from build123d import *

# Parameters (mm, degrees)
SKETCH1_W               = 100
SKETCH1_H               = 70
BOSS_EXTRUDE1_DEPTH     = 6
SKETCH2_W               = 100
SKETCH2_H               = 6
BOSS_EXTRUDE2_DEPTH     = 50
CUT_EXTRUDE1_DEPTH      = 103.645019363
CUT_EXTRUDE1_DEPTH_BACK = 103.645019363
SKETCH3_R               = 1.5
SKETCH3_R_2             = 2
CUT_EXTRUDE2_DEPTH      = 103.645019363
CUT_EXTRUDE2_DEPTH_BACK = 103.645019363
CUT_EXTRUDE3_DEPTH      = 103.645019363
CUT_EXTRUDE4_DEPTH      = 103.645019363
CUT_EXTRUDE4_DEPTH_BACK = 103.645019363
CUT_EXTRUDE5_DEPTH      = 103.645019363
CUT_EXTRUDE5_DEPTH_BACK = 103.645019363
SKETCH9_W               = 15
SKETCH9_H               = 3.5
BOSS_EXTRUDE3_DEPTH     = 10
CUT_EXTRUDE8_START      = -3.5
SKETCH11_R              = 2
CUT_EXTRUDE8_DEPTH      = 12
FILLET1_R               = 5
FILLET2_R               = 5
FILLET3_R               = 5
FILLET4_R               = 5
CUT_EXTRUDE9_DEPTH      = 103.645019363
SKETCH14_R              = 5
CUT_EXTRUDE10_DEPTH     = 3
CUT_EXTRUDE11_START     = -3
SKETCH15_R              = 5
CUT_EXTRUDE11_DEPTH     = 3
SKETCH16_R              = 5
CUT_EXTRUDE12_DEPTH     = 3
CUT_EXTRUDE13_START     = -3
SKETCH17_R              = 5
CUT_EXTRUDE13_DEPTH     = 3


with BuildPart() as part:
    # Sketch1 → Boss-Extrude1 (new body)
    with BuildSketch(Plane(origin=(0, 0, 0), x_dir=(1, 0, 0), z_dir=(0, 1, 0))):
        Rectangle(SKETCH1_W, SKETCH1_H)
    extrude(amount=BOSS_EXTRUDE1_DEPTH)

    # Sketch2 → Boss-Extrude2 (add)
    with BuildSketch(Plane(origin=(0, 6, 0), x_dir=(1, 0, 0), z_dir=(0, 1, 0))):
        with Locations((0, 32)):
            Rectangle(SKETCH2_W, SKETCH2_H)
        with Locations((0, -32)):
            Rectangle(SKETCH2_W, SKETCH2_H)
    extrude(amount=BOSS_EXTRUDE2_DEPTH)

    # Sketch3 → Cut-Extrude1 (cut, two sides: drawn at the far end of the back side and taken through both)
    with BuildSketch(Plane.XY.offset(35).offset(-CUT_EXTRUDE1_DEPTH_BACK)):
        with Locations((-35, 11)):
            Circle(SKETCH3_R)
        with Locations((25, 11)):
            Circle(SKETCH3_R_2)
    extrude(amount=CUT_EXTRUDE1_DEPTH + CUT_EXTRUDE1_DEPTH_BACK, mode=Mode.SUBTRACT)

    # Sketch4 → Cut-Extrude2 (cut, two sides: drawn at the far end of the back side and taken through both)
    with BuildSketch(Plane.XY.offset(35).offset(-CUT_EXTRUDE2_DEPTH_BACK)):
        Polygon((-50, 25), (3.693575035, 56), (-50, 56), align=None)
    extrude(amount=CUT_EXTRUDE2_DEPTH + CUT_EXTRUDE2_DEPTH_BACK, mode=Mode.SUBTRACT)

    # Sketch5 → Cut-Extrude3 (cut, through all)
    with BuildSketch(Plane.XY.offset(35)):
        Polygon((26.846787517, 56), (50, 28), (50, 56), align=None)
    extrude(amount=-CUT_EXTRUDE3_DEPTH, mode=Mode.SUBTRACT)

    # Sketch6 → Cut-Extrude4 (cut, two sides: drawn at the far end of the back side and taken through both)
    with BuildSketch(Plane.XY.offset(35).offset(-CUT_EXTRUDE4_DEPTH_BACK)):
        Polygon((16.600357162, 47.527222171), (39.753569645, 19.527222171), (47.460108019, 25.899762189), (24.306895537, 53.899762189), align=None)
    extrude(amount=CUT_EXTRUDE4_DEPTH + CUT_EXTRUDE4_DEPTH_BACK, mode=Mode.SUBTRACT)

    # Sketch7 → Cut-Extrude5 (cut, two sides: drawn at the far end of the back side and taken through both)
    with BuildSketch(Plane.XY.offset(35).offset(-CUT_EXTRUDE5_DEPTH_BACK)):
        Polygon((2.673241004, 38.01310693), (-4.304705141, 32.243040152), (11.948586847, 12.587358417), (18.926532993, 18.357425196), align=None)
        Polygon((-15.212346405, 34.449406206), (-22.19029255, 28.679339427), (-9.445212514, 13.266262678), (-2.467266369, 19.036329456), align=None)
    extrude(amount=CUT_EXTRUDE5_DEPTH + CUT_EXTRUDE5_DEPTH_BACK, mode=Mode.SUBTRACT)

    # Sketch9 → Boss-Extrude3 (add)
    with BuildSketch(Plane(origin=(0, 6, 0), x_dir=(1, 0, 0), z_dir=(0, 1, 0))):
        with Locations((-17.5, 4.25)):
            Rectangle(SKETCH9_W, SKETCH9_H)
        with Locations((-17.5, -4.25)):
            Rectangle(SKETCH9_W, SKETCH9_H)
    extrude(amount=BOSS_EXTRUDE3_DEPTH)

    # Sketch11 → Cut-Extrude8 (cut)
    with BuildSketch(Plane.XY.offset(-2.5).offset(CUT_EXTRUDE8_START)):
        with Locations((-17.5, 11)):
            Circle(SKETCH11_R)
    extrude(amount=CUT_EXTRUDE8_DEPTH, mode=Mode.SUBTRACT)

    # Fillet1
    fillet1_edges = [part.edges().sort_by_distance(p)[0] for p in [
        (-25, 16, -4.25),
    ]]
    fillet(fillet1_edges, radius=FILLET1_R)

    # Fillet2
    fillet2_edges = [part.edges().sort_by_distance(p)[0] for p in [
        (-10, 16, -4.25),
    ]]
    fillet(fillet2_edges, radius=FILLET2_R)

    # Fillet3
    fillet3_edges = [part.edges().sort_by_distance(p)[0] for p in [
        (-25, 16, 4.25),
    ]]
    fillet(fillet3_edges, radius=FILLET3_R)

    # Fillet4
    fillet4_edges = [part.edges().sort_by_distance(p)[0] for p in [
        (-10, 16, 4.25),
    ]]
    fillet(fillet4_edges, radius=FILLET4_R)

    # Sketch13 → Cut-Extrude9 (cut, through all)
    with BuildSketch(Plane(origin=(0, 0, -35), x_dir=(-1, 0, 0), z_dir=(0, 0, -1))):
        Polygon((-50, 12), (-39.487682116, 12), (-11.373066959, 46), (13.626933041, 46), (-3.693575035, 56), (-26.846787517, 56), (-50, 28), align=None)
    extrude(amount=-CUT_EXTRUDE9_DEPTH, mode=Mode.SUBTRACT)

    # Sketch14 → Cut-Extrude10 (cut)
    with BuildSketch(Plane.XY.offset(35)):
        with Locations((25, 11)):
            Circle(SKETCH14_R)
    extrude(amount=-CUT_EXTRUDE10_DEPTH, mode=Mode.SUBTRACT)

    # Sketch15 → Cut-Extrude11 (cut)
    with BuildSketch(Plane(origin=(0, 0, -35), x_dir=(-1, 0, 0), z_dir=(0, 0, -1)).offset(CUT_EXTRUDE11_START)):
        with Locations(Location((-25, 11, 0), (0, 0, 180))):
            Circle(SKETCH15_R)
    extrude(amount=CUT_EXTRUDE11_DEPTH, mode=Mode.SUBTRACT)

    # Sketch16 → Cut-Extrude12 (cut)
    with BuildSketch(Plane(origin=(0, 0, -35), x_dir=(-1, 0, 0), z_dir=(0, 0, -1))):
        with Locations((35, 11)):
            Circle(SKETCH16_R)
    extrude(amount=-CUT_EXTRUDE12_DEPTH, mode=Mode.SUBTRACT)

    # Sketch17 → Cut-Extrude13 (cut)
    with BuildSketch(Plane.XY.offset(35).offset(CUT_EXTRUDE13_START)):
        with Locations(Location((-35, 11, 0), (0, 0, 180))):
            Circle(SKETCH17_R)
    extrude(amount=CUT_EXTRUDE13_DEPTH, mode=Mode.SUBTRACT)


solid = part.part
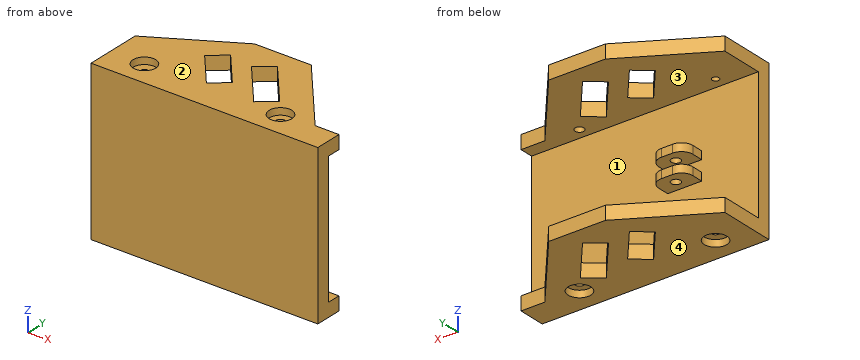
Here's how the part is built. I have some questions about the finished solid (model axes, mm). Face numbers are marked on the shaded views. Coordinates: 2 decimals unless noted, no trailing zeros. Write each loop counter-clockwise with the first axis right and the second up, starting at its lowest first coordinate (ties: lowest second). Pieces come first, ordered by that corner, then holes.
Item 1: I want a section at C-C on x = 13. Write out the boundary of the cut face in (y, z).
Item 2: If I drill on line 1 (X direction, y = 11, z = 30.15); line 2 (Z direction, x = 21, y = 32); line 3 (Z direction, x = 24, y = 9), over which ranges is the centre line in solid material (lowest first)?
Item 3: I want a section at D-D on x = 43. Write out the boundary of the cut face in (y, z).
Item 4: If we mould it in two halves opening along Z, with no side actions, what happens to the marked faces 1, 2, 3 and 4? For each: +Z half, -Z half, draft (parallel to the pull), parting line (faces both ways), or undercut.
Item 5: I want a section at A-A on x = -17.5. Count the separate pieces of the cut face and the enclosed holes in it, and give its area (3 significant figures).
Item 6: I want a section at B-B on y = 36.5. Write out the boundary of the cut face in (x, z).
Item 7: Will these pins go through, and if not, where does the flat tip stop? pin 1 (13 mm diameter, centred on x = -35, y = 11, fed in from -Z); pin 2 (4 mm diameter, centred on y = 9, z = 3.5, fed in from +X); pin 3 (1 mm diameter, centred on x = -17, z = 4.5, fed in from +Y); pin 4 (4 mm diameter, centred on y = 9.5, z = -4.5, fed in from -X).
Findings below:
1. outline: (0, -35) - (13.46, -35) - (13.46, -29) - (6, -29) - (6, 29) - (13.46, 29) - (13.46, 35) - (0, 35) - close; (25.52, -35) - (44.03, -35) - (44.03, -29) - (25.52, -29) - close; (25.52, 29) - (44.03, 29) - (44.03, 35) - (25.52, 35) - close
2. line 1: x = -50 to -36.5, -33.5 to 23, 27 to 50
2. line 2: z = -35 to -29, 29 to 35
2. line 3: z = -32 to -29, 29 to 32
3. outline: (0, -35) - (12, -35) - (12, -29) - (6, -29) - (6, 29) - (12, 29) - (12, 35) - (0, 35) - close
4. face 1: undercut
4. face 2: +Z half
4. face 3: undercut
4. face 4: -Z half
5. separate pieces: 5
5. enclosed holes: 0
5. area: 801 mm2
6. outline: (-30.08, -35) - (0.84, -35) - (0.84, -29) - (-30.08, -29) - close; (-30.08, 29) - (0.84, 29) - (0.84, 35) - (-30.08, 35) - close; (3.92, -35) - (19.23, -35) - (19.23, -29) - (3.92, -29) - close; (3.92, 29) - (19.23, 29) - (19.23, 35) - (3.92, 35) - close
7. pin 1: stops at z = -35
7. pin 2: stops at x = -10
7. pin 3: stops at y = 16
7. pin 4: stops at x = -25
